```python
from build123d import *

# Parameters (mm, degrees)
F0_R     = 3.05
F1_DEPTH = 11.25
F2_DEPTH = 2.25
F4_D     = 2
F4_DEPTH = 25.501
F5_D     = 2


with BuildPart() as f1:
    # F0 (on Top) → F1 (new body)
    with BuildSketch(Plane.XY):
        with BuildLine():
            Line((7.9630808905, -0.7676866104), (7.9630808905, 0.7676866104))
            ThreePointArc((7.9630808905, 0.7676866104), (6.5707016234, 4.5635381204), (3.5, 7.193747285))
            Line((3.5, 7.193747285), (3.5, -7.193747285))
            ThreePointArc((3.5, -7.193747285), (6.5707016234, -4.5635381204), (7.9630808905, -0.7676866104))
        make_face()
        with BuildLine():
            Line((3.5, -7.193747285), (3.5, 7.193747285))
            ThreePointArc((3.5, 7.193747285), (0, 8), (-3.5, 7.193747285))
            Line((-3.5, 7.193747285), (-3.5, -7.193747285))
            ThreePointArc((-3.5, -7.193747285), (0, -8), (3.5, -7.193747285))
        make_face()
        Circle(F0_R, mode=Mode.SUBTRACT)
        with BuildLine():
            Line((-3.5, -7.193747285), (-3.5, 7.193747285))
            ThreePointArc((-3.5, 7.193747285), (-6.5707016234, 4.5635381204), (-7.9630808905, 0.7676866104))
            Line((-7.9630808905, 0.7676866104), (-7.9630808905, -0.7676866104))
            ThreePointArc((-7.9630808905, -0.7676866104), (-6.5707016234, -4.5635381204), (-3.5, -7.193747285))
        make_face()
        with BuildLine():
            Line((-3.5, 13.5), (-3.5, 25.2586618806))
            ThreePointArc((-3.5, 25.2586618806), (-5.7548058579, 24.842145832), (-7.9630808905, 24.2247671347))
            Line((-7.9630808905, 24.2247671347), (-7.9630808905, 13.5))
            Line((-7.9630808905, 13.5), (-3.5, 13.5))
        make_face()
        with BuildLine():
            Line((7.9630808905, 13.5), (7.9630808905, 24.2247671347))
            ThreePointArc((7.9630808905, 24.2247671347), (5.7548058579, 24.842145832), (3.5, 25.2586618806))
            Line((3.5, 25.2586618806), (3.5, 13.5))
            Line((3.5, 13.5), (7.9630808905, 13.5))
        make_face()
        with BuildLine():
            ThreePointArc((3.5, -25.2586618806), (5.7548058579, -24.842145832), (7.9630808905, -24.2247671347))
            Line((7.9630808905, -24.2247671347), (7.9630808905, -13.5))
            Line((7.9630808905, -13.5), (3.5, -13.5))
            Line((3.5, -13.5), (3.5, -25.2586618806))
        make_face()
        with BuildLine():
            ThreePointArc((-7.9630808905, -24.2247671347), (-5.7548058579, -24.842145832), (-3.5, -25.2586618806))
            Line((-3.5, -25.2586618806), (-3.5, -13.5))
            Line((-3.5, -13.5), (-7.9630808905, -13.5))
            Line((-7.9630808905, -13.5), (-7.9630808905, -24.2247671347))
        make_face()
        with BuildLine():
            Line((-3.5, 7.193747285), (-3.5, 13.5))
            Line((-3.5, 13.5), (-7.9630808905, 13.5))
            Line((-7.9630808905, 13.5), (-7.9630808905, 3))
            Line((-7.9630808905, 3), (-7.9630808905, 0.7676866104))
            ThreePointArc((-7.9630808905, 0.7676866104), (-6.5707016234, 4.5635381204), (-3.5, 7.193747285))
        make_face()
        with BuildLine():
            Line((7.9630808905, 0.7676866104), (7.9630808905, 3))
            Line((7.9630808905, 3), (7.9630808905, 13.5))
            Line((7.9630808905, 13.5), (3.5, 13.5))
            Line((3.5, 13.5), (3.5, 7.193747285))
            ThreePointArc((3.5, 7.193747285), (6.5707016234, 4.5635381204), (7.9630808905, 0.7676866104))
        make_face()
        with BuildLine():
            Line((7.9630808905, -13.5), (7.9630808905, -3))
            Line((7.9630808905, -3), (7.9630808905, -0.7676866104))
            ThreePointArc((7.9630808905, -0.7676866104), (6.5707016234, -4.5635381204), (3.5, -7.193747285))
            Line((3.5, -7.193747285), (3.5, -13.5))
            Line((3.5, -13.5), (7.9630808905, -13.5))
        make_face()
        with BuildLine():
            Line((-7.9630808905, -13.5), (-3.5, -13.5))
            Line((-3.5, -13.5), (-3.5, -7.193747285))
            ThreePointArc((-3.5, -7.193747285), (-6.5707016234, -4.5635381204), (-7.9630808905, -0.7676866104))
            Line((-7.9630808905, -0.7676866104), (-7.9630808905, -3))
            Line((-7.9630808905, -3), (-7.9630808905, -13.5))
        make_face()
        with BuildLine():
            Line((-7.9630808905, 3), (-25.3229145242, 3))
            ThreePointArc((-25.3229145242, 3), (-25.5, 0), (-25.3229145242, -3))
            Line((-25.3229145242, -3), (-7.9630808905, -3))
            Line((-7.9630808905, -3), (-7.9630808905, -0.7676866104))
            ThreePointArc((-7.9630808905, -0.7676866104), (-8, 0), (-7.9630808905, 0.7676866104))
            Line((-7.9630808905, 0.7676866104), (-7.9630808905, 3))
        make_face()
        with BuildLine():
            ThreePointArc((25.3229145242, -3), (25.4556901337, -1.5026109997), (25.5, 0))
            ThreePointArc((25.5, 0), (25.4556901337, 1.5026109997), (25.3229145242, 3))
            Line((25.3229145242, 3), (7.9630808905, 3))
            Line((7.9630808905, 3), (7.9630808905, 0.7676866104))
            ThreePointArc((7.9630808905, 0.7676866104), (7.9907648922, 0.3842869216), (8, 0))
            ThreePointArc((8, 0), (7.9907648922, -0.3842869216), (7.9630808905, -0.7676866104))
            Line((7.9630808905, -0.7676866104), (7.9630808905, -3))
            Line((7.9630808905, -3), (25.3229145242, -3))
        make_face()
        with BuildLine():
            Line((-3.5, -13.5), (3.5, -13.5))
            Line((3.5, -13.5), (3.5, -7.193747285))
            ThreePointArc((3.5, -7.193747285), (0, -8), (-3.5, -7.193747285))
            Line((-3.5, -7.193747285), (-3.5, -13.5))
        make_face()
        with BuildLine():
            Line((3.5, 7.193747285), (3.5, 13.5))
            Line((3.5, 13.5), (-3.5, 13.5))
            Line((-3.5, 13.5), (-3.5, 7.193747285))
            ThreePointArc((-3.5, 7.193747285), (0, 8), (3.5, 7.193747285))
        make_face()
    extrude(amount=F1_DEPTH)

    # F0 (on Top) → F2 (join)
    with BuildSketch(Plane.XY):
        with BuildLine():
            ThreePointArc((-25.3229145242, -3), (-19.7385931025, -16.1442851292), (-7.9630808905, -24.2247671347))
            Line((-7.9630808905, -24.2247671347), (-7.9630808905, -13.5))
            Line((-7.9630808905, -13.5), (-7.9630808905, -3))
            Line((-7.9630808905, -3), (-25.3229145242, -3))
        make_face()
        with BuildLine():
            Line((-3.5, -13.5), (3.5, -13.5))
            Line((3.5, -13.5), (3.5, -7.193747285))
            ThreePointArc((3.5, -7.193747285), (0, -8), (-3.5, -7.193747285))
            Line((-3.5, -7.193747285), (-3.5, -13.5))
        make_face()
        with BuildLine():
            Line((3.5, 7.193747285), (3.5, 13.5))
            Line((3.5, 13.5), (-3.5, 13.5))
            Line((-3.5, 13.5), (-3.5, 7.193747285))
            ThreePointArc((-3.5, 7.193747285), (0, 8), (3.5, 7.193747285))
        make_face()
        with BuildLine():
            ThreePointArc((7.9630808905, -24.2247671347), (19.7385931025, -16.1442851292), (25.3229145242, -3))
            Line((25.3229145242, -3), (7.9630808905, -3))
            Line((7.9630808905, -3), (7.9630808905, -13.5))
            Line((7.9630808905, -13.5), (7.9630808905, -24.2247671347))
        make_face()
        with BuildLine():
            Line((7.9630808905, 3), (25.3229145242, 3))
            ThreePointArc((25.3229145242, 3), (19.7385931025, 16.1442851292), (7.9630808905, 24.2247671347))
            Line((7.9630808905, 24.2247671347), (7.9630808905, 13.5))
            Line((7.9630808905, 13.5), (7.9630808905, 3))
        make_face()
        with BuildLine():
            Line((-7.9630808905, 13.5), (-7.9630808905, 24.2247671347))
            ThreePointArc((-7.9630808905, 24.2247671347), (-19.7385931025, 16.1442851292), (-25.3229145242, 3))
            Line((-25.3229145242, 3), (-7.9630808905, 3))
            Line((-7.9630808905, 3), (-7.9630808905, 13.5))
        make_face()
    extrude(amount=F2_DEPTH)

    # F4 (through all, one way)
    with BuildSketch(Plane.YZ):
        with Locations((-19.5, 4.75), (19.5, 4.75)):
            Circle(F4_D / 2)
    extrude(amount=-F4_DEPTH, mode=Mode.SUBTRACT)

    # F5 (through all)
    with Locations(Plane(origin=(0, 0, 0), x_dir=(0, 1, 0), z_dir=(-1, 0, 0))):
        with Locations((-19.5, -4.75), (19.5, -4.75)):
            Hole(F5_D / 2)


solid = f1.part
```
CAD build for the part. Positions are in the model's coordinates, mm. A direction names the side the tool comes from. Coordinates: 2 decimals unless noted, no trailing zeros. Write each loop counter-clockwise with the first axis right and the second up, starting at its lowest first coordinate (ties: lowest second). Pieces come first, ordered by that corner, then holes.
(1) Cut at C-C, the plane x = -1.5. List the corners of the cut face in (y, z).
(2) Drill centre lines: probe 1 along X at (y, z) = (-22, 5.75); probe 2 along Y at (x, z) = (5.7, 4.75); probe 3 along Y at (x, z) = (-4.9, 4.75). Where is each one in solid material? Low to high.
(3) Cut at B-B, the plane y = -19.5. List the corners of the cut face in (x, z), and give its area (3 significant figures).
(4) Cut at D-D, the plane z = 4.75. Count the separate pieces of the cut face and the enclosed holes in it, and give its area (3 significant figures).
(5) 3-axis set-ups, long thin cutter, end or side, ignore diameter. For faces 4 (the face through (-3.5, -19, 7)), 5 (the face through (-17, -3, 7)), 6 (the face through (17, -3, 7)), 7 (the face through (17, 3, 7)), 8 (the face through (-7.963, 14, 7)): which of +Z, -Z, +X, -X, +Y, -Y reach the whole face in a straight line?
(6) Two-plate mould, pull along Z, no slides. Class faces 1 (the face through (3.5, 19, 7)), 2 (the face through (5.8, 20.5, 4.7)), 3 (the face through (15, -11, 2.25)): +Z half, -Z half, draft (parallel to the pull), parting line (faces both ways), or undercut.
(7) Cut at A-A, the plane z = 8.5. List the corners of the cut face in (x, y).
(8) Flat gauge pins, fed straight in: pin 1 (2 mm diameter, centred on x = -20, y = -10, fed in from +Z); pin 2 (2.5 mm diameter, centred on y = 19.5, z = 4.75, fed in from +X); pin 3 (1.8 mm diameter, centred on y = -19.5, z = 4.75, fed in from +X); pin 4 (4.5 mm diameter, centred on y = 10.5, z = 5.5, fed in from -X). Where does each tip first touch, or does it go through?
Geometry says:
1. outline: (-13.5, 0) - (-2.66, 0) - (-2.66, 11.25) - (-13.5, 11.25) - close; (2.66, 0) - (13.5, 0) - (13.5, 11.25) - (2.66, 11.25) - close
2. probe 1: x = -7.96 to -3.5, 3.5 to 7.96
2. probe 2: y = -24.85 to -20.5, -18.5 to 18.5, 20.5 to 24.85
2. probe 3: y = -25.02 to -20.5, -18.5 to 18.5, 20.5 to 25.02
3. outline: (-16.43, 0) - (-3.5, 0) - (-3.5, 3.75) - (-7.96, 3.75) - (-7.96, 2.25) - (-16.43, 2.25) - close; (-7.96, 5.75) - (-3.5, 5.75) - (-3.5, 11.25) - (-7.96, 11.25) - close; (3.5, 0) - (16.43, 0) - (16.43, 2.25) - (7.96, 2.25) - (7.96, 3.75) - (3.5, 3.75) - close; (3.5, 5.75) - (7.96, 5.75) - (7.96, 11.25) - (3.5, 11.25) - close
3. area: 121 mm2
4. separate pieces: 5
4. enclosed holes: 3
4. area: 777 mm2
5. face 4: +Z, -Z, -Y
5. face 5: +Z, -X, -Y
5. face 6: +Z, +X, -Y
5. face 7: +Z, +X, +Y
5. face 8: +Z, -X, +Y
6. face 1: draft
6. face 2: undercut
6. face 3: +Z half
7. outline: (-25.32, -3) - (-7.96, -3) - (-7.96, -24.22) arc R25.5 ccw to (-3.5, -25.26) - (-3.5, -13.5) - (3.5, -13.5) - (3.5, -25.26) arc R25.5 ccw to (7.96, -24.22) - (7.96, -3) - (25.32, -3) arc R25.5 ccw to (25.32, 3) - (7.96, 3) - (7.96, 24.22) arc R25.5 ccw to (3.5, 25.26) - (3.5, 13.5) - (-3.5, 13.5) - (-3.5, 25.26) arc R25.5 ccw to (-7.96, 24.22) - (-7.96, 3) - (-25.32, 3) arc R25.5 ccw to start; hole (-7.96, -0.77) - (-7.96, 0.77) arc R8 ccw to start; hole circle Ø6.1 at (0, 0); hole (7.96, -0.77) arc R8 ccw to (7.96, 0.77) - close
8. pin 1: stops at z = 2.25
8. pin 2: stops at x = 7.96
8. pin 3: passes through
8. pin 4: stops at x = -7.96
